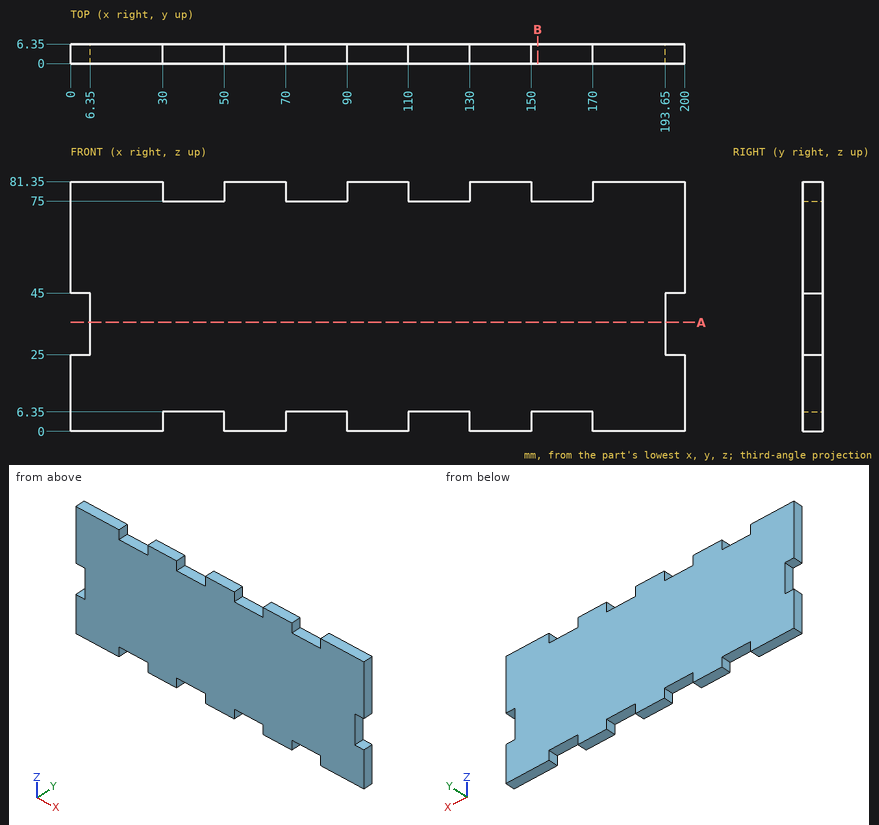
Check sheet for the drawn part. Datum: minimum x, y, z corner. Units: mm. Give positions to 0.01 mm unless a question says otherwise; leave off trailing zeros. Order: outer loops, then holes, each group sorted by start corner. A loop starts at its lowest first (then second) coordinate and runs counter-clockwise, first axis right, second up. Notation, with made-up numbers: (42.5, 32) - (86.5, 32) arc R27 ccw to (86.5, 49) - close; hole circle Ø8 at (83.5, -27). An arc over 180 degrees is marked (long way). Answer in a Markdown table with one row per item. Add a question column.
Q1. Gauge pin test, flat end, axial feed: pin 1 (3 mm diameter, centred on y = 2.5, z = 40, fed in from -X). Record the tip position at first contact, or that the pin passes through.
Q2. Cross-section at B-B, the plane x = 152. Enter the section's corners in (y, z), then the cut area to 3 significant figures.
Q3. Cross-section at A-A, the plane z = 35.5. Enter the section's corners in (x, y), then the cut area to 3 significant figures.
Q4. Material ranges on probe 1 along X at (y, z) = (3, 76); probe 2 along X at (y, z) = (5.5, 31.5); probe 3 along Z at (x, y) = (113, 2), recorded low to high. Write a range as from..to.
Check values:
| question | item | result |
|---|---|---|
| 1 | pin 1 | stops at x = 6.35 |
| 2 | outline | (0, 6.35) - (6.35, 6.35) - (6.35, 75) - (0, 75) - close |
| 2 | area | 436 mm^2 |
| 3 | outline | (6.35, 0) - (193.65, 0) - (193.65, 6.35) - (6.35, 6.35) - close |
| 3 | area | 1,190 mm^2 |
| 4 | probe 1 | x = 0..30, 50..70, 90..110, 130..150, 170..200 |
| 4 | probe 2 | x = 6.35..193.65 |
| 4 | probe 3 | z = 6.35..75 |
